Autodesk Inventor part; units mm, degrees
ref_plane "YZ Plane" through (0, 0, 0) normal (1, 0, 0) x (0, 1, 0)
ref_plane "XZ Plane" through (0, 0, 0) normal (0, 1, 0) x (-1, 0, 0)
sketch "Sketch3" plane through (0, 0, 0) normal (0, 0, 1) x (1, 0, 0)
  line L0 (0, -9.525) -> (9.525, -9.525)
  line L1 (9.525, -9.525) -> (9.525, 0)
  line L2 (0, 0) -> (0, -9.525) construction
  line L3 (0, 0) -> (9.525, 0) construction
  line L4 (0, -9.525) -> (-9.525, -9.525)
  line L5 (-9.525, -9.525) -> (-9.525, 0)
  line L6 (9.525, 0) -> (73.025, 0)
  line L7 (-187.325, 0) -> (-187.325, 19.05)
  line L8 (-187.325, 0) -> (-9.525, 0)
  line L9 (73.025, 0) -> (73.025, 19.05)
  line L10 (73.025, 19.05) -> (-187.325, 19.05)
  dimension "d0" = 9.525
  dimension "d1" = 9.525
  dimension "d6" = 63.5
  dimension "d8" = 19.05
  dimension "d9" = 177.8
extrude "Extrusion1" add sketch "Sketch3" along normal mid plane 355.6
sketch "Sketch4" plane through (0, 0, 177.8) normal (0, 0, 1) x (1, 0, 0)
  line L0 (-187.325, 19.05) -> (73.025, 19.05) construction
  line L1 (0, 19.05) -> (0, -9.525) construction
  line L2 (9.525, -9.525) -> (-9.525, -9.525) construction
  line L3 (0, -9.525) -> (-22.225, -9.525)
  line L4 (-22.225, -9.525) -> (-22.225, 19.05)
  line L5 (-22.225, 19.05) -> (0, 19.05)
  line L6 (187.325, 19.05) -> (-73.025, 19.05) construction
  line L7 (0, -9.525) -> (22.225, -9.525)
  line L8 (22.225, -9.525) -> (22.225, 19.05)
  line L9 (0, 19.05) -> (22.225, 19.05)
  point P0 (0, 0)
  dimension "d12" = 22.225
extrude "Extrusion2" add sketch "Sketch4" along normal blind 12.7
mirror "Mirror1" about plane through (0, 0, 0) normal (0, 0, 1) of "Extrusion2"
sketch "Sketch6" plane through (-187.325, 0, -177.8) normal (0, -1, 0) x (1, 0, 0)
  line L0 (82.55, 165.1) -> (88.9, 165.1)
  line L1 (88.9, 165.1) -> (88.9, 190.5)
  line L2 (88.9, 190.5) -> (82.55, 190.5)
  line L3 (82.55, 190.5) -> (82.55, 165.1)
  line L4 (82.55, 165.1) -> (88.9, 190.5) construction
  line L5 (88.9, 165.1) -> (82.55, 190.5) construction
  line L6 (177.8, 0) -> (177.8, 355.6)
  point P0 (187.325, 177.8)
  point P1 (85.725, 177.8)
  dimension "d16" = 12.7
  dimension "d18" = 6.35
  dimension "d19" = 88.9
extrude "Extrusion3" cut sketch "Sketch6" against normal through all
sketch "Sketch7" plane through (0, 0, 177.8) normal (0, 0, 1) x (1, 0, 0)
  line L0 (-187.325, 19.05) -> (-22.225, 19.05)
  line L1 (-161.925, 19.05) -> (-117.475, 19.05)
  line L2 (-117.475, 19.05) -> (-117.475, -3.81)
  line L3 (-117.475, -3.81) -> (-161.925, -3.81)
  line L4 (-161.925, -3.81) -> (-161.925, 19.05)
  line L5 (-187.325, 19.05) -> (-187.325, 0)
  point P0 (0, 0)
  dimension "d22" = 44.45
  dimension "d23" = 22.86
  dimension "d24" = 25.4
extrude "Extrusion4" add sketch "Sketch7" along normal blind 12.7
mirror "Mirror2" about plane through (0, 0, 0) normal (0, 0, 1) of "Extrusion4"
sketch "Sketch9" plane through (73.025, 0, 177.8) normal (1, 0, 0) x (0, 0, -1)
  line L0 (355.6, 19.05) -> (0, 19.05)
  line L1 (50.8, 19.05) -> (63.5, 19.05)
  line L2 (63.5, 19.05) -> (63.5, 12.7)
  line L3 (63.5, 12.7) -> (50.8, 12.7)
  line L4 (50.8, 12.7) -> (50.8, 19.05)
  line L5 (0, 0) -> (0, 19.05)
  point P0 (177.8, 0)
  dimension "d28" = 12.7
  dimension "d29" = 6.35
  dimension "d30" = 50.8
extrude "Extrusion5" cut sketch "Sketch9" against normal through all
mirror "Mirror3" about plane through (0, 0, 0) normal (0, 0, 1) of "Extrusion5"
sketch "Sketch12" plane through (73.025, 0, 177.8) normal (1, 0, 0) x (0, 0, -1)
  line L0 (355.6, 0) -> (0, 0) construction
  line L1 (88.9, 0) -> (88.9, 16.5009) construction
  line L2 (0, 0) -> (0, 19.05)
  line L3 (50.8, 19.05) -> (0, 19.05)
  line L4 (84.1375, 19.05) -> (84.1375, 12.7)
  line L5 (84.1375, 12.7) -> (80.1624, 12.7)
  line L6 (80.1624, 12.7) -> (80.1624, 6.35)
  line L7 (80.1624, 6.35) -> (88.9, 6.35)
  line L8 (93.6625, 19.05) -> (93.6625, 12.7)
  line L9 (93.6625, 12.7) -> (97.6376, 12.7)
  line L10 (97.6376, 12.7) -> (97.6376, 6.35)
  line L11 (97.6376, 6.35) -> (88.9, 6.35)
  line L12 (84.1375, 19.05) -> (93.6625, 19.05)
  point P0 (177.8, 0)
  dimension "d46" = 88.9
  dimension "d47" = 4.7625
  dimension "d48" = 6.35
  dimension "d49" = 6.35
  dimension "d50" = 8.7376
extrude "Extrusion8" cut sketch "Sketch12" against normal through all
mirror "Mirror4" about plane through (0, 0, 0) normal (0, 0, 1) of "Extrusion8"
split "Split2" plane through (0, 0, 0) removes the side toward (0, 0, -1)
ref_plane "Work Plane1" through (-60.325, 0, 177.8) normal (1, 0, 0) x (0, 0, -1)
split "Split3" plane through (-60.325, 0, 177.8) removes the side toward (-1, 0, 0)
properties part number "BandSawJigBottomSpiltA-SpiltA" material "LCP Plastic"
Part model, mm, in its own coordinate system. A direction names the side the tool comes from. Round coordinates to 2 decimals unless told otherwise and drop trailing zeros. Write each loop counter-clockwise with the first axis right and the second up, starting at its lowest first coordinate (ties: lowest second). Pieces come first, ordered by that corner, then holes. Notation, with made-up numbers: (19.25, -3.75) -> (32.25, -3.75) arc R37 ccw to (32.25, 33.25) -> close; hole circle Ø11 at (80, 78.5). An arc over 180 degrees is marked (long way). Return JSON: item names as keys, results as strings. Group by question number.
Q1. Saw through at B-B on z = 76. Write the cut outline in (x, y) (3 decimals), plus the area to 3 significant figures.
Q2. Saw through at D-D on y = -2.5. Write the cut outline in (x, z) (3 decimals), plus the area to 3 significant figures.
Q3. Probe L1, parallel to Z at x = 36, y = 15; L2, parallel to Z at x = -48, y = 7; L3, parallel to Z at x = -5.5, y = 14.5. List the from-to ranges inside material, lowest first. Write a range as [from, to].
Q4. Saw through at A-A on y = 17. Write the cut outline in (x, z) (1 decimal), plus the area to 3 significant figures.
Q5. Mould opens along Y. For faces 1 (the flat face through (7, 12.7, 82)), 2 (the flat face through (7, 6.35, 89)), 3 (the flat face through (22.225, 5, 184)), 4 (the flat face through (-35, 0, 88)) say: pulls with the +Y half, pulls with the -Y half, needs draft (parallel to the pull), parting line crosses it, or undercut.
Q6. Which spindle directions (+Z, -Z, +X, -X, +Y, -Y) get a long thin tool onto all of the face, cutting with end or side? Do faces 5 (the flat face through (16, -5, 177.8)), 6 (the flat face through (-9.525, -5, 88)), 7 (the flat face through (7, 16, 93.662)). Say none if no direction does.
Q7. Pin check, flat tips, straight feed: pin 1 (5 mm diameter, centred on x = -16, z = 91.5, fed in from -Y); pin 2 (5 mm diameter, centred on y = -5, z = 116, fed in from +X) (3 decimals); pin 3 (7.5 mm diameter, centred on x = 14, y = -4.5, fed in from -Z). Stop position of each tip, or through.
Q8. Saw through at C-C on x = -42. Write the cut outline in (y, z), plus the area to 4 significant figures.
Answer:
{
 "1": {"outline": "(-60.325, 0) -> (-9.525, 0) -> (-9.525, -9.525) -> (9.525, -9.525) -> (9.525, 0) -> (73.025, 0) -> (73.025, 19.05) -> (-60.325, 19.05) -> close", "area": "2,720 mm2"},
 "2": {"outline": "(-22.225, 177.8) -> (-9.525, 177.8) -> (-9.525, 0) -> (9.525, 0) -> (9.525, 177.8) -> (22.225, 177.8) -> (22.225, 190.5) -> (-22.225, 190.5) -> close", "area": "3,950 mm2"},
 "3": {"L1": "[0, 84.14], [93.66, 114.3], [127, 177.8]", "L2": "[0, 80.16], [97.64, 177.8]", "L3": "[0, 84.14], [93.66, 114.3], [127, 190.5]"},
 "4": {"outline": "(-60.3, 0) -> (73, 0) -> (73, 84.1) -> (-60.3, 84.1) -> close; (-60.3, 93.7) -> (73, 93.7) -> (73, 114.3) -> (-60.3, 114.3) -> close; (-60.3, 127) -> (73, 127) -> (73, 177.8) -> (22.2, 177.8) -> (22.2, 190.5) -> (-22.2, 190.5) -> (-22.2, 177.8) -> (-60.3, 177.8) -> close", "area": "21,300 mm2"},
 "5": {"face 1": "undercut", "face 2": "undercut", "face 3": "needs draft", "face 4": "pulls with the -Y half"},
 "6": {"face 5": "-Z, +X, -Y", "face 6": "-Z, -X, -Y", "face 7": "+X, -X, +Y"},
 "7": {"pin 1": "y = 0", "pin 2": "x = 9.525", "pin 3": "z = 177.8"},
 "8": {"outline": "(0, 0) -> (19.05, 0) -> (19.05, 84.14) -> (12.7, 84.14) -> (12.7, 80.16) -> (6.35, 80.16) -> (6.35, 97.64) -> (12.7, 97.64) -> (12.7, 93.66) -> (19.05, 93.66) -> (19.05, 114.3) -> (12.7, 114.3) -> (12.7, 127) -> (19.05, 127) -> (19.05, 177.8) -> (0, 177.8) -> close", "area": "3,135 mm2"}
}
